The figure shows three views and two pictorial views of one solid part (mm, origin at its lowest corner). Answer the questions. Give positions to 0.01 mm unless a question says otherwise; leave off trailing zeros. Loops run counter-clockwise (first coordinate to the right, second up) from the corner with the lowest first, then second, coordinate; pieces in that order, holes last. Notation, with made-up numbers: (51, 83.5) - (67, 83.5) arc R14 cw to (67, 99.5) - close; hole circle Ø8 at (-25.75, 45). An arc over 180 degrees is marked (long way). Use a Markdown table: item, result. Add a question column.
Item 1: A cutting plane is placed at B-B (z = 141.5). Determine the outline of the cut face in (x, y).
Item 2: Each of these flat-tipped pins is pushed along its axis until it touches: P1, Ø2.5, axis at x = 39, z = 45, coming from the -Y side; P2, Ø1.8, axis at x = 10, z = 25, coming from the +Y side. Where does it stop, or does it pass through?
Item 3: Consider probe 1 along Z at (x, y) = (16, 1.95); probe 2 along X at (y, z) = (3.6, 165); probe 3 along Z at (x, y) = (10, 3.25). Determine where each line is inside the solid, lowest interval first. Write a range as [from, to].
Item 4: A cutting plane is placed at A-A (y = 1.45). Give the number of separate pieces and of enclosed holes in the cut face, plus the area to 3 significant figures.
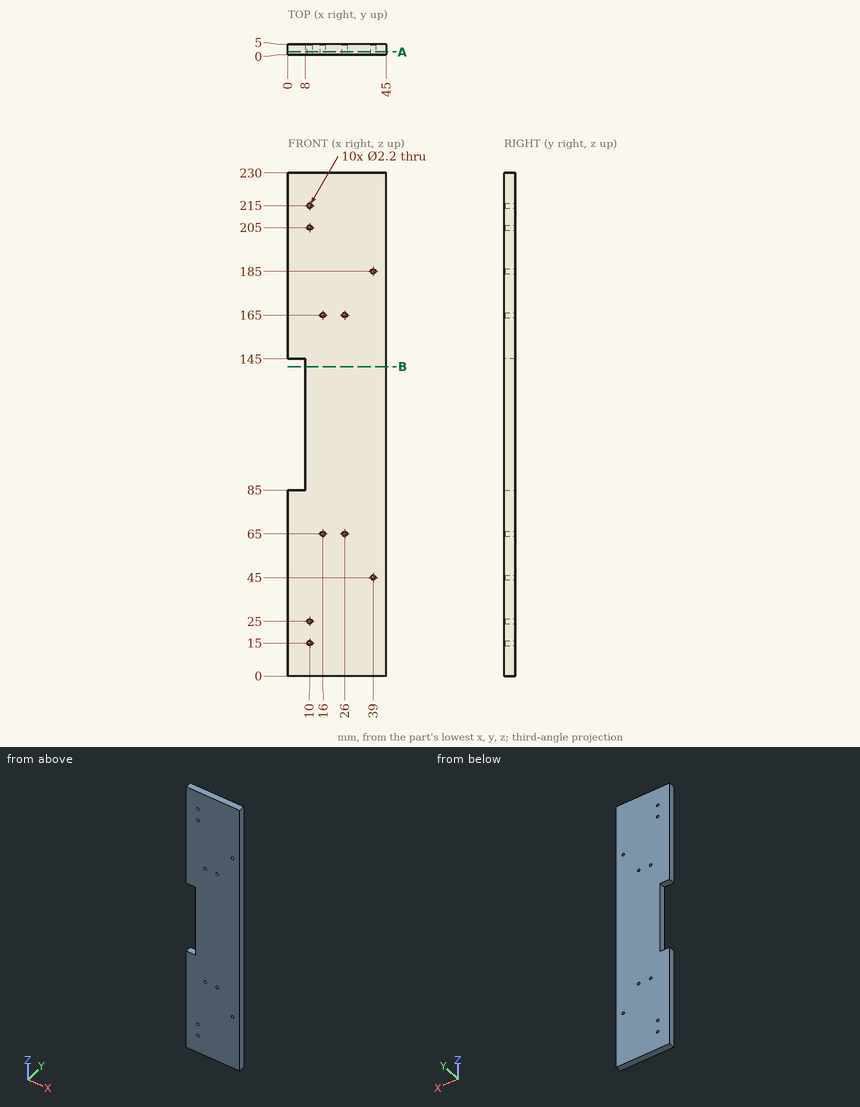
Geometry says:
| question | item | result |
|---|---|---|
| 1 | outline | (8, 0) - (45, 0) - (45, 5) - (8, 5) - close |
| 2 | P1 | y = 0 |
| 2 | P2 | through |
| 3 | probe 1 | [0, 63.9], [66.1, 163.9], [166.1, 230] |
| 3 | probe 2 | [0, 14.9], [17.1, 24.9], [27.1, 45] |
| 3 | probe 3 | [0, 13.9], [16.1, 23.9], [26.1, 203.9], [206.1, 213.9], [216.1, 230] |
| 4 | separate pieces | 1 |
| 4 | enclosed holes | 10 |
| 4 | area | 9,830 mm² |
